Autodesk Fusion 360 part; units mm, degrees
sketch "Sketch1" plane through (0, 0, 0) normal (1, 0, 0) x (0, 1, 0)
  circle A0 centre (0, 0) radius 5
  circle A1 centre (0, 0) radius 0.5
  dimension "d1" = 10
  dimension "d2" = 1
extrude "Extrude1" add sketch "Sketch1" along normal blind 23 contours A0 | A1
extrude "Extrude2" add sketch "Sketch1" against normal blind 1 contours A1
fillet "Fillet1" radius 1 2 edges at (0, -4.6616, -1.8081) (23, -4.6616, -1.8081)
sketch "Sketch2" plane through (0, 0, 0) normal (0, 0, 1) x (1, 0, 0)
  line L0 (0, 15) -> (0, -10) construction
  line L1 (11.5, 15) -> (11.5, -7) construction
  line L2 (-5, 0) -> (27.3814, 0) construction
  line L3 (9.5, 2) -> (13.5, 2)
  line L4 (13.5, 2) -> (13.5, -2)
  line L5 (13.5, -2) -> (9.5, -2)
  line L6 (9.5, -2) -> (9.5, 2)
  line L7 (9.5, 2) -> (13.5, -2) construction
  line L8 (13.5, 2) -> (9.5, -2) construction
  point P0 (11.5, 0)
  dimension "d9" = 11.5
  dimension "d10" = 4
  dimension "d11" = 4
extrude "Extrude3" cut sketch "Sketch2" along normal blind 5
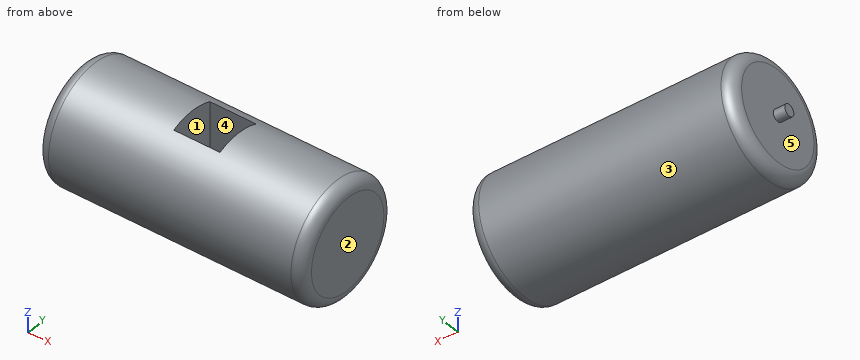
Geometry check sheet. Reference: the model listing, model coordinates, mm. Face numbers are marked on the shaded views. A direction names the side the tool comes from. Round coordinates to 2 decimals unless told otherwise and drop trailing zeros. Order: outer loops, then holes, each group sorted by start corner. A loop starts at its lowest first (then second) coordinate and runs counter-clockwise, first axis right, second up. Notation, with made-up numbers: (-39, 30.25) - (-26, 30.25) arc R36 ccw to (-26, 65.25) - close; hole circle Ø10 at (-10, 75.5). An arc over 180 degrees is marked (long way). Use a Markdown table: item, result. Add a question column.
1) Gauge pin test, flat ends, axial feed: P1, Ø2, axis at x = 12, z = 1.5, coming from the +Y side; P2, Ø3, axis at x = 3, z = -3, coming from the -Y side; P3, Ø1.2, axis at x = 12, z = 1.5, coming from the -Y side. Record the tip position at first contact, or that the pin passes through.
2) Mould release check, pull along Y, two halves, no side actions. Record for the marked faces 3, 4 and 5: released by +Y, released by -Y, zero draft, split by the parting line, or undercut.
3) Section check B-B (x = 1.5). Record the cut outline in (y, z), then the cut area to 3 significant figures.
4) Set-up check for the marked faces 1 and 2: record each of +Z, -Z, +X, -X, +Y, -Y from which the full face is reachable in a straight line by a thin tool's end or side.
5) Section check A-A (y = 0). Record the cut outline in (x, z), then the cut area to 3 significant figures.
6) Thickness scan on line 1 along X through (y, z) = (1.25, 0.5); line 2 along X through (y, z) = (-2, -1.25); line 3 along Y through (x, z) = (12.25, 3.5). Record the ranges inside material, lowest first.
Established:
| question | item | result |
|---|---|---|
| 1 | P1 | y = 4.97 |
| 1 | P2 | y = -4.77 |
| 1 | P3 | y = -4.92 |
| 2 | face 3 | split by the parting line |
| 2 | face 4 | undercut |
| 2 | face 5 | zero draft |
| 3 | outline | circle Ø10 at (0, 0) |
| 3 | area | 78.5 mm2 |
| 4 | face 1 | +Z |
| 4 | face 2 | +Z, -Z, +X, +Y, -Y |
| 5 | outline | (-1, -0.5) - (0, -0.5) - (0, -4) arc R1 ccw to (1, -5) - (22, -5) arc R1 ccw to (23, -4) - (23, 4) arc R1 ccw to (22, 5) - (13.5, 5) - (13.5, 0) - (9.5, 0) - (9.5, 5) - (1, 5) arc R1 ccw to (0, 4) - (0, 0.5) - (-1, 0.5) - close |
| 5 | area | 210 mm2 |
| 6 | line 1 | 0 to 9.5, 13.5 to 23 |
| 6 | line 2 | 0 to 23 |
| 6 | line 3 | -3.57 to -2, 2 to 3.57 |
